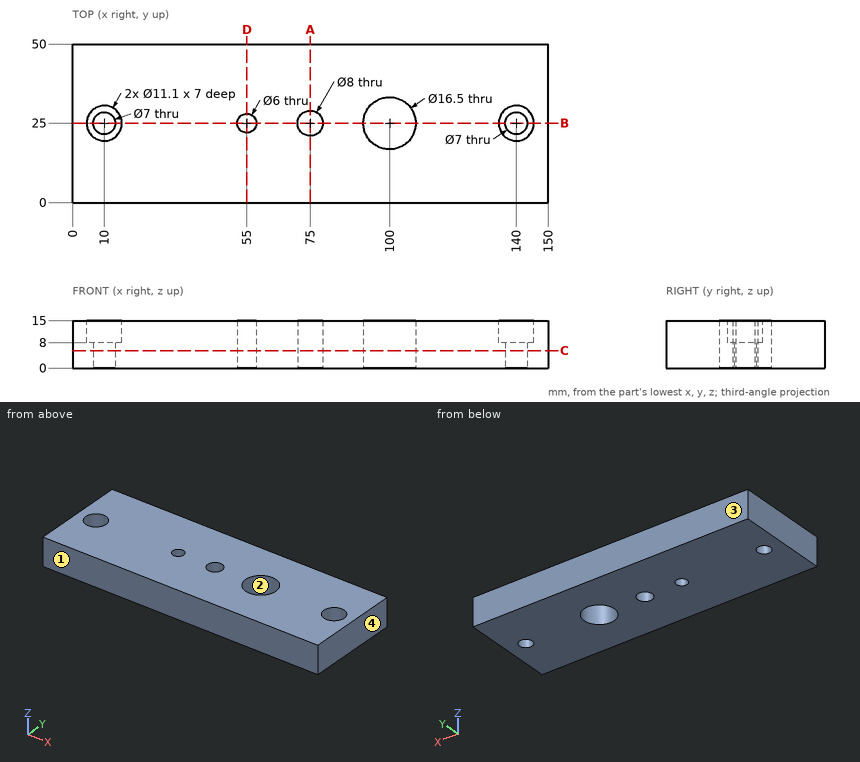
Design review of the part shown in the three views and the two pictorial views. Dimensions are in mm from the part's minimum x, y and z. Round coordinates to 2 decimals unless told otherwise and drop trailing zeros. Write each loop counter-clockwise with the first axis right and the second up, starting at its lowest first coordinate (ties: lowest second). Pieces come first, ordered by that corner, then holes. Notation, with made-up numbers: (-15.75, 43) - (25.25, 43) arc R37 ccw to (25.25, 80) - close; hole circle Ø6 at (76.25, -13). An arc over 180 degrees is marked (long way). Write item = value, one per line. Start each with the question number.
1. Consider section D-D on x = 55. State the section outline as (y, z) points, plus the area to 3 significant figures.
2. Consider section A-A on x = 75. State the section outline as (y, z) points.
3. Draft analysis for pull direction Y (two halves, no side actions). For the marked faces 1, 2, 3 and 4, state which applies: released by +Y, released by -Y, zero draft, split by the parting line, or undercut.
4. Wall thickness on L1, parallel to Y at x = 140, z = 5.5; L2, parallel to Y at x = 10, z = 10.25; L3, parallel to X at y = 30, z = 12.75: over which ranges is each line inside the solid? List them lowest first.
5. For pin 1 Ø3.5 at (x, y) = (142, 25.5) entering from +Z; pin 2 Ø19 at (x, y) = (100, 25) entering from +Z, all flat-tipped, find the tip position at first contact; note any pin that passes through.
6. Consider section B-B on y = 25. Give the number of separate pieces and of enclosed holes in the cut face, plus the area to 3 significant figures.
7. Consider section C-C on z = 5.5. State the section outline as (x, y) points, plus the area to 3 significant figures.
Evaluation:
q1.outline = (0, 0) - (22, 0) - (22, 15) - (0, 15) - close; (28, 0) - (50, 0) - (50, 15) - (28, 15) - close
q1.area = 660 mm2
q2.outline = (0, 0) - (21, 0) - (21, 15) - (0, 15) - close; (29, 0) - (50, 0) - (50, 15) - (29, 15) - close
q3.face_1 = released by -Y
q3.face_2 = undercut
q3.face_3 = released by +Y
q3.face_4 = zero draft
q4.L1 = 0 to 21.5, 28.5 to 50
q4.L2 = 0 to 19.45, 30.55 to 50
q4.L3 = 0 to 7.59, 12.41 to 93.44, 106.56 to 137.59, 142.41 to 150
q5.pin_1 = 8
q5.pin_2 = 15
q6.separate_pieces = 6
q6.enclosed_holes = 0
q6.area = 1,530 mm2
q7.outline = (0, 0) - (150, 0) - (150, 50) - (0, 50) - close; hole circle Ø7 at (10, 25); hole circle Ø6 at (55, 25); hole circle Ø8 at (75, 25); hole circle Ø16.5 at (100, 25); hole circle Ø7 at (140, 25)
q7.area = 7,130 mm2
